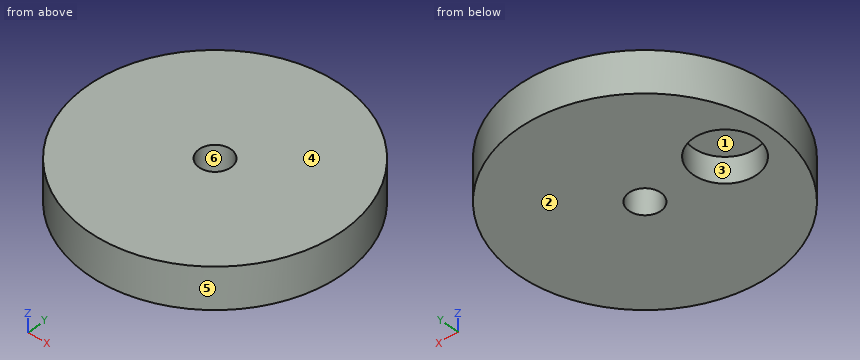
from build123d import *

# Parameters (mm, degrees)
F0_R     = 40
F0_R_2   = 10
F0_R_3   = 5
F1_DEPTH = 5
F2_DEPTH = 8


with BuildPart() as f1:
    # F0 (on Top) → F1 (new body)
    with BuildSketch(Plane.XY):
        Circle(F0_R)
        with Locations((-25, 0)):
            Circle(F0_R_2, mode=Mode.SUBTRACT)
        Circle(F0_R_3, mode=Mode.SUBTRACT)
        with Locations((-25, 0)):
            Circle(F0_R_2)
    extrude(amount=F1_DEPTH)

    # F0 (on Top) → F2 (join)
    with BuildSketch(Plane.XY):
        Circle(F0_R)
        with Locations((-25, 0)):
            Circle(F0_R_2, mode=Mode.SUBTRACT)
        Circle(F0_R_3, mode=Mode.SUBTRACT)
    extrude(amount=-F2_DEPTH)


solid = f1.part
Geometry check sheet. Reference: the model listing, model coordinates, mm. Face numbers are marked on the shaded views. A direction names the side the tool comes from. Coordinates: 2 decimals unless noted, no trailing zeros. Order: outer loops, then holes, each group sorted by start corner. A loop starts at its lowest first (then second) coordinate and runs counter-clockwise, first axis right, second up. Notation, with made-up numbers: (58, 44.25) -> (75, 44.25) arc R32 cw to (75, 76.25) -> close; hole circle Ø6 at (-20, 41). An arc over 180 degrees is marked (long way). Use a Markdown table: item, result. Add a question column.
1. Cross-section at A-A (y = 0). Enter the section's corners in (x, z).
2. Go/stop test with flat-tipped pins: pin 1 Ø2 at (x, z) = (14, -0.5) entering from -Y; pin 2 Ø16 at (x, y) = (-25, 0) entering from -Z; pin 3 Ø2 at (y, z) = (-30, -1) entering from +X; pin 4 Ø6 at (x, y) = (0, 0) entering from -Z. Record where each tip stops, or that it passes through.
3. Set-up check for the marked faces 1 and 2: record each of +Z, -Z, +X, -X, +Y, -Y from which the full face is reachable in a straight line by a thin tool's end or side.
4. Cross-section at D-D (z = 1.75). Enter the section's corners in (x, y).
5. Mould release check, pull along Y, two halves, no side actions. Record for the marked faces 3, 4, 5 and 6: pulls with the +Y half, pulls with the -Y half, needs draft (parallel to the pull), parting line crosses it, or undercut.
6. Material ranges on L1, parallel to X at y = -4, z = -6.75; L2, parallel to Y at x = 0, z = 0.5; L3, parallel to X at y = -2.5, z = -7, recorded low to high.
7. Cross-section at B-B (x = 0). Enter the section's corners in (y, z), and give its area (3 significant figures).
8. Cross-section at C-C (z = -2.75). Enter the section's corners in (x, y).
Filled sheet:
| question | item | result |
|---|---|---|
| 1 | outline | (-40, -8) -> (-35, -8) -> (-35, 0) -> (-15, 0) -> (-15, -8) -> (-5, -8) -> (-5, 5) -> (-40, 5) -> close; (5, -8) -> (40, -8) -> (40, 5) -> (5, 5) -> close |
| 2 | pin 1 | y = -37.83 |
| 2 | pin 2 | z = 0 |
| 2 | pin 3 | x = 27.55 |
| 2 | pin 4 | through |
| 3 | face 1 | -Z |
| 3 | face 2 | -Z, +X, -X, +Y, -Y |
| 4 | outline | circle Ø80 at (0, 0); hole circle Ø10 at (0, 0) |
| 5 | face 3 | undercut |
| 5 | face 4 | needs draft |
| 5 | face 5 | parting line crosses it |
| 5 | face 6 | undercut |
| 6 | L1 | -39.8 to -34.17, -15.83 to -3, 3 to 39.8 |
| 6 | L2 | -40 to -5, 5 to 40 |
| 6 | L3 | -39.92 to -34.68, -15.32 to -4.33, 4.33 to 39.92 |
| 7 | outline | (-40, -8) -> (-5, -8) -> (-5, 5) -> (-40, 5) -> close; (5, -8) -> (40, -8) -> (40, 5) -> (5, 5) -> close |
| 7 | area | 910 mm2 |
| 8 | outline | circle Ø80 at (0, 0); hole circle Ø20 at (-25, 0); hole circle Ø10 at (0, 0) |
